Can you work these out from the model? Positions are in its coordinate system, mm. Round coordinates to 2 decimals unless told otherwise and drop trailing zeros. Order: outer loops, then holes, each group sorted by start corner. A loop starts at its lowest first (then second) coordinate and runs counter-clockwise, first axis right, second up. Notation, with made-up numbers: (5, -19.5) -> (29, -19.5) arc R33 ccw to (29, 19.5) -> close; hole circle Ø8 at (-25, 41). An arc over 180 degrees is marked (long way). Use a Markdown table: item, result. Add a question column.
Q1. I need wall thicknesses on line 1 along Z through (x, y) = (194.5, 103); line 2 along X through (y, z) = (44, 2.3); line 3 along X through (y, z) = (48, 2.65). Which ranges of each line are inside material? Lowest first, please. Write a range as [from, to].
Q2. If we section it at D-D on y = 30: List the corners of the cut face in (x, z) for me (1 decimal).
Q3. If we section it at A-A on y = 100.5: List the corners of the cut face in (x, z) for me (1 decimal), plus the area to 3 significant figures.
Q4. If we section it at C-C on x = 280: List the corners of the cut face in (y, z) for me (1 decimal).
Q5. If we section it at B-B on x = 68: List the corners of the cut face in (y, z) for me (1 decimal), plus the area to 3 significant figures.
```python
from build123d import *

# Parameters (mm, degrees)
BOSS_EXTRUDE1_DEPTH = 4.7625
CHAMFER1_SIZE       = 1.5875
CHAMFER1_SIZE2      = 12.7
CHAMFER2_SIZE       = 1.5875
CHAMFER2_SIZE2      = 12.7
BOSS_EXTRUDE2_DEPTH = 4.445


with BuildPart() as part:
    # Sketch1 → Boss-Extrude1 (new body)
    with BuildSketch(Plane.XY):
        Polygon((0, 0), (457.2, 0), (381, 177.8), (304.8, 177.8), align=None)
    extrude(amount=BOSS_EXTRUDE1_DEPTH)

    # Chamfer1
    chamfer1_edges = [part.edges().sort_by_distance(p)[0] for p in [
        (152.4, 88.9, 4.7625),
        (152.4, 88.9, 0),
    ]]
    chamfer1_side = [part.faces().sort_by_distance(p)[0] for p in [
        (152.4, 88.9, 2.38125),
    ]]
    chamfer(chamfer1_edges, length=CHAMFER1_SIZE, length2=CHAMFER1_SIZE2, reference=chamfer1_side[0])

    # Chamfer2
    chamfer2_edges = [part.edges().sort_by_distance(p)[0] for p in [
        (419.1, 88.9, 4.7625),
        (419.1, 88.9, 0),
    ]]
    chamfer2_side = [part.faces().sort_by_distance(p)[0] for p in [
        (419.1, 88.9, 2.38125),
    ]]
    chamfer(chamfer2_edges, length=CHAMFER2_SIZE, length2=CHAMFER2_SIZE2, reference=chamfer2_side[0])

    # Sketch2 → Boss-Extrude2 (add)
    with BuildSketch(Plane.XZ):
        Polygon((25.204862667, 0), (443.382811651, 0), (457.2, 1.5875), (457.2, 3.175), (443.382811651, 4.7625), (25.204862667, 4.7625), (0, 3.175), (0, 1.5875), align=None)
    extrude(amount=BOSS_EXTRUDE2_DEPTH)


solid = part.part
```
Answer below:
| question | item | result |
|---|---|---|
| 1 | line 1 | [0.46, 4.3] |
| 1 | line 2 | [75.43, 438.34] |
| 1 | line 3 | [82.29, 436.63] |
| 2 | outline | (51.4, 1.6) -> (76.6, 0) -> (430.5, 0) -> (444.3, 1.6) -> (444.3, 3.2) -> (430.5, 4.8) -> (76.6, 4.8) -> (51.4, 3.2) -> close |
| 3 | outline | (172.3, 1.6) -> (197.5, 0) -> (400.3, 0) -> (414.1, 1.6) -> (414.1, 3.2) -> (400.3, 4.8) -> (197.5, 4.8) -> (172.3, 3.2) -> close |
| 3 | area | 1,090 mm² |
| 4 | outline | (-4.4, 0) -> (148.6, 0) -> (163.3, 1.6) -> (163.3, 3.2) -> (148.6, 4.8) -> (-4.4, 4.8) -> close |
| 5 | outline | (-4.4, 0) -> (25, 0) -> (39.7, 1.6) -> (39.7, 3.2) -> (25, 4.8) -> (-4.4, 4.8) -> close |
| 5 | area | 187 mm² |
